from build123d import *

# Parameters (mm, degrees)
F1_DEPTH = 3.175
F2_R     = 1.5875
F3_R     = 2.249995
F4_DEPTH = 3.176
F5_R     = 3.96875
F5_W     = 11.1125
F5_H     = 3.175
F6_DEPTH = 3.176


with BuildPart() as f1:
    # F0 (on Top) → F1 (new body)
    with BuildSketch(Plane.XY):
        with BuildLine():
            Line((25.4, 34.925), (-25.4, 34.925))
            ThreePointArc((-25.4, 34.925), (-27.645064, 33.995064), (-28.575, 31.75))
            Line((-28.575, 31.75), (-28.575, -31.75))
            ThreePointArc((-28.575, -31.75), (-27.645064, -33.995064), (-25.4, -34.925))
            Line((-25.4, -34.925), (25.4, -34.925))
            ThreePointArc((25.4, -34.925), (27.645064, -33.995064), (28.575, -31.75))
            Line((28.575, -31.75), (28.575, 31.75))
            ThreePointArc((28.575, 31.75), (27.645064, 33.995064), (25.4, 34.925))
        make_face()
    extrude(amount=F1_DEPTH)

    # F2
    f2_edges = [f1.edges().sort_by_distance(p)[0] for p in [
        (0, -34.925, 3.175),
        (-28.575, 0, 3.175),
    ]]
    fillet(f2_edges, radius=F2_R)

    # F3 (on face) → F4 (cut, through all)
    with BuildSketch(Plane.XY.offset(3.175)):
        with Locations((-25.4, 31.75)):
            Circle(F3_R)
        with Locations((25.4, 31.75)):
            Circle(F3_R)
        with Locations((25.4, -31.75)):
            Circle(F3_R)
        with Locations((-25.4, -31.75)):
            Circle(F3_R)
    extrude(amount=-F4_DEPTH, mode=Mode.SUBTRACT)

    # F5 (on face) → F6 (cut, through all)
    with BuildSketch(Plane.XY.offset(3.175)):
        with Locations((-14.2875, -6.985)):
            Circle(F5_R)
        with Locations((-14.2875, 6.985)):
            Circle(F5_R)
        with Locations((-14.2875, 20.955)):
            Circle(F5_R)
        with Locations((0, 29.059681)):
            Rectangle(F5_W, F5_H)
    extrude(amount=-F6_DEPTH, mode=Mode.SUBTRACT)


solid = f1.part
Source: CAD feature listing. Evaluate the final solid. Frame: model axes, mm. A direction names the side the tool comes from. Give positions to 0.01 mm unless a question says otherwise; leave off trailing zeros. Loops run counter-clockwise (first coordinate to the right, second up) from the corner with the lowest first, then second, coordinate; pieces in that order, holes last. Notation, with made-up numbers: (3, -29.75) -> (26, -29.75) arc R35 ccw to (26, 7.25) -> close; hole circle Ø4 at (26, 44.5). An arc over 180 degrees is marked (long way). Use a Markdown table: item, result. Add a question column.
1) Reachability of faces 5 (the face through (0, 27.472, 2)), 6 (the face through (28.12, 0.44, 2.7)) from +Z, -Z, +X, -X, +Y, -Y: full face, straight path, thin tool, end or side. Return the list, or none.
2) Line query: line 1 along X through (y, z) = (31.75, 1.55) (3 decimals); line 2 along X through (y, z) = (-30, 1.7); line 3 along Y through (x, z) = (25.4, 1.95). Output: solid intervals per line, ascending. Write a range as [from, to].
3) Section query A-A, the plane y = 8.5. Return the cut outline in (x, z) (1 decimal), then the cut area to 3 significant figures.
4) Pull-direction query (Y, two-part tool) for faces 1 (the face through (27.62, -34.02, 0.78)), 2 (the face through (0, 30.647, 2)), 3 (the face through (-0.36, 34.47, 2.7)), 4 (the face through (-28.575, 0, 1)); classes: +Y half, -Y half, draft (parallel to the pull), parting line (faces both ways), or undercut.
5) Section query B-B, the plane x = -2. Return the cut outline in (y, z) (1 decimal), then the cut area to 3 significant figures.
6) Section query C-C, the plane x = -17. Return the cut outline in (y, z) (1 decimal), then the cut area to 3 significant figures.
7) Section query D-D, the plane z = 2.4. Count the separate pieces of the cut face and the enclosed holes in it, then the cut area to 3 significant figures.
Numbers:
| question | item | result |
|---|---|---|
| 1 | face 5 | +Z, -Z |
| 1 | face 6 | +Z, +X, +Y, -Y |
| 2 | line 1 | x = [-28.575, -27.65], [-23.15, 23.15], [27.65, 28.575] |
| 2 | line 2 | x = [-28.57, -26.81], [-23.99, 23.99], [26.81, 28.57] |
| 2 | line 3 | y = [-34.88, -34], [-29.5, 29.5], [34, 34.88] |
| 3 | outline | (-28.6, 0) -> (-18, 0) -> (-18, 3.2) -> (-27, 3.2) arc R1.6 ccw to (-28.6, 1.6) -> close; (-10.6, 0) -> (28.6, 0) -> (28.6, 1.6) arc R1.6 ccw to (27, 3.2) -> (-10.6, 3.2) -> close |
| 3 | area | 157 mm2 |
| 4 | face 1 | -Y half |
| 4 | face 2 | undercut |
| 4 | face 3 | +Y half |
| 4 | face 4 | draft |
| 5 | outline | (-34.9, 0) -> (27.5, 0) -> (27.5, 3.2) -> (-33.3, 3.2) arc R1.6 ccw to (-34.9, 1.6) -> close; (30.6, 0) -> (34.9, 0) -> (34.9, 1.6) arc R1.6 ccw to (33.3, 3.2) -> (30.6, 3.2) -> close |
| 5 | area | 211 mm2 |
| 6 | outline | (-34.9, 0) -> (-9.9, 0) -> (-9.9, 3.2) -> (-33.3, 3.2) arc R1.6 ccw to (-34.9, 1.6) -> close; (-4.1, 0) -> (4.1, 0) -> (4.1, 3.2) -> (-4.1, 3.2) -> close; (9.9, 0) -> (18.1, 0) -> (18.1, 3.2) -> (9.9, 3.2) -> close; (23.9, 0) -> (34.9, 0) -> (34.9, 1.6) arc R1.6 ccw to (33.3, 3.2) -> (23.9, 3.2) -> close |
| 6 | area | 166 mm2 |
| 7 | separate pieces | 1 |
| 7 | enclosed holes | 8 |
| 7 | area | 3,680 mm2 |
